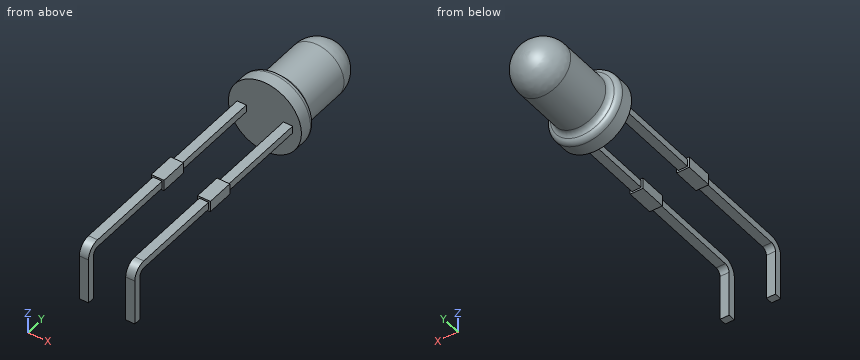
```python
from build123d import *

# Parameters (mm, degrees)
FILLET_1_R      = 0.3
FILLET_2_R      = 0.3
SKETCH_2_W      = 0.5
SKETCH_2_H      = 0.4
EXTRUDE_1_DEPTH = 5
SKETCH_3_W      = 0.7
SKETCH_3_H      = 0.6
EXTRUDE_2_DEPTH = 1.5
SKETCH_5_W      = 0.5
SKETCH_5_H      = 0.4
EXTRUDE_3_DEPTH = 4.5
SWEEP_START     = -1.52
SWEEP_2_DEPTH   = 0.5
SKETCH_7_262_W  = 0.5
SKETCH_7_262_H  = 0.4


# Read off the part's stored shape, not the designer's step: По траектории2
with BuildPart() as part:
    # Эскиз1 → Повернуть2 (revolve)
    with BuildSketch(Plane(origin=(0, 0, 0), x_dir=(0, 0, -1), z_dir=(1, 0, 0))):
        with BuildLine():
            Line((0, 0), (-2, 0))
            Line((-2, 0), (-2, 1))
            Line((-2, 1), (-1.5, 1))
            Line((-1.5, 1), (-1.5, 4))
            ThreePointArc((-1.5, 4), (-1.07971355, 5.07971355), (0, 5.5))
            Line((0, 5.5), (0, 0))
        make_face()
    revolve(axis=Axis((0, 5.5, 0), (0, -1, 0)))

    # Скругление1
    fillet_1_edges = [part.edges().sort_by_distance(p)[0] for p in [
        (0, 1, -2),
    ]]
    fillet(fillet_1_edges, radius=FILLET_1_R)

    # Скругление2
    fillet_2_edges = [part.edges().sort_by_distance(p)[0] for p in [
        (0, 1, -1.5),
    ]]
    fillet(fillet_2_edges, radius=FILLET_2_R)

    # Эскиз2 → Вытянуть1 (add)
    with BuildSketch(Plane.XZ):
        with Locations((-1.27, 0)):
            Rectangle(SKETCH_2_W, SKETCH_2_H)
        with Locations((1.27, 0)):
            Rectangle(SKETCH_2_W, SKETCH_2_H)
    extrude(amount=EXTRUDE_1_DEPTH)

    # Эскиз3 → Вытянуть2 (add)
    with BuildSketch(Plane.XZ.offset(5)):
        with Locations((-1.27, 0)):
            Rectangle(SKETCH_3_W, SKETCH_3_H)
        with Locations((1.27, 0)):
            Rectangle(SKETCH_3_W, SKETCH_3_H)
    extrude(amount=EXTRUDE_2_DEPTH)

    # Эскиз5 → Вытянуть3 (add)
    with BuildSketch(Plane.XZ.offset(6.5)):
        with Locations((-1.27, 0)):
            Rectangle(SKETCH_5_W, SKETCH_5_H)
        with Locations((1.27, 0)):
            Rectangle(SKETCH_5_W, SKETCH_5_H)
    extrude(amount=EXTRUDE_3_DEPTH)

    # По траектории2 outline → По траектории2 (add)
    with BuildSketch(Plane.YZ.offset(SWEEP_START)):
        with BuildLine():
            Line((-11.5, -0.2), (-11, -0.2))
            Line((-11, -0.2), (-11, 0.2))
            Line((-11, 0.2), (-11.5, 0.2))
            ThreePointArc((-11.5, 0.2), (-11.994974747, -0.005025253), (-12.2, -0.5))
            Line((-12.2, -0.5), (-12.2, -3))
            Line((-12.2, -3), (-11.8, -3))
            Line((-11.8, -3), (-11.8, -0.5))
            ThreePointArc((-11.8, -0.5), (-11.712132034, -0.287867966), (-11.5, -0.2))
        make_face()
    extrude(amount=SWEEP_2_DEPTH)

    # По траектории11: sweep along a curve in space
    with BuildLine() as sweep_11_path:
        Line((-1.27, -11, 0), (-1.27, -11.5, 0))
        ThreePointArc((-1.27, -11.5, 0), (-1.27, -11.853553391, -0.146446609), (-1.27, -12, -0.5))
        Line((-1.27, -12, -0.5), (-1.27, -12, -3))
    # Эскиз7<262> → По траектории11 (sweep)
    with BuildSketch(Plane.XZ.offset(11)):
        with Locations((-1.27, 0)):
            Rectangle(SKETCH_7_262_W, SKETCH_7_262_H)
        with Locations((1.27, 0)):
            Rectangle(SKETCH_7_262_W, SKETCH_7_262_H)
    sweep(path=sweep_11_path.line)


solid = part.part
```
The listing builds one solid part. Answer for the finished solid, in the listing's coordinates (mm). Give positions to 0.01 mm unless a question says otherwise; leave off trailing zeros. Order: outer loops, then holes, each group sorted by start corner. A loop starts at its lowest first (then second) coordinate and runs counter-clockwise, first axis right, second up. Notation, with made-up numbers: (-12.5, 42.25) -> (21.5, 42.25) arc R30 ccw to (21.5, 75.25) -> close; hole circle Ø2 at (79, 16). An arc over 180 degrees is marked (long way). Answer as a JSON object with one key per item and string values. Group by question number.
Item 1: The part is cut by section A-A on y = -10.75. Write down the section's boundary in (x, z).
Item 2: The part is cut by section B-B on y = 1.75. Write down the section's boundary in (x, z), and give its area (3 significant figures).
Item 3: Flat-ended cylindrical pins translate along their axes: pin 1 (3 mm diameter, centred on y = -5, z = 0.5, fed in from +X); pin 2 (1.5 mm diameter, centred on x = 1.5, y = -8.5, fed in from +Z). Find the tip coordinate at first contact, or state that the pin passes through.
Item 4: Consider L1, parallel to X at y = -1.75, z = 0; L2, parallel to Z at x = -1.1, y = 3.5; L3, parallel to X at y = 3.25, z = 1.3. Determine where each line is inside the solid, lowest interval first. Write a range as from..to.
Result set:
{
 "1": {"outline": "(-1.52, -0.2) -> (-1.02, -0.2) -> (-1.02, 0.2) -> (-1.52, 0.2) -> close; (1.02, -0.2) -> (1.52, -0.2) -> (1.52, 0.2) -> (1.02, 0.2) -> close"},
 "2": {"outline": "circle Ø3 at (0, 0)", "area": "7.07 mm²"},
 "3": {"pin 1": "x = 1.62", "pin 2": "z = 0.2"},
 "4": {"L1": "-1.52..-1.02, 1.02..1.52", "L2": "-1.02..1.02", "L3": "-0.75..0.75"}
}
